```python
from build123d import *

# Parameters (mm, degrees)
SKETCH1_W           = 70
SKETCH1_H           = 50
BOSS_EXTRUDE1_DEPTH = 50
SKETCH2_W           = 20
SKETCH2_H           = 10
CUT_EXTRUDE1_DEPTH  = 50
CUT_EXTRUDE2_DEPTH  = 50
CUT_EXTRUDE3_DEPTH  = 30
SKETCH6_W           = 10
SKETCH6_H           = 10
CUT_EXTRUDE4_DEPTH  = 10
BOSS_EXTRUDE2_DEPTH = 10
CUT_EXTRUDE5_DEPTH  = 10
BOSS_EXTRUDE3_DEPTH = 10
BOSS_EXTRUDE4_DEPTH = 10
BOSS_EXTRUDE5_DEPTH = 10
BOSS_EXTRUDE6_DEPTH = 22


with BuildPart() as part:
    # Sketch1 → Boss-Extrude1 (new body)
    with BuildSketch(Plane.XY):
        with Locations((35, 25)):
            Rectangle(SKETCH1_W, SKETCH1_H)
    extrude(amount=BOSS_EXTRUDE1_DEPTH)

    # Sketch2 → Cut-Extrude1 (cut)
    with BuildSketch(Plane.XY.offset(50)):
        Polygon((0, 20), (30, 50), (0, 50), align=None)
        with Locations((60, 45)):
            Rectangle(SKETCH2_W, SKETCH2_H)
    extrude(amount=-CUT_EXTRUDE1_DEPTH, mode=Mode.SUBTRACT)

    # Sketch3 → Cut-Extrude2 (cut)
    with BuildSketch(Plane.XZ):
        Polygon((0, 10), (20, 20), (20, 50), (0, 50), align=None)
    extrude(amount=-CUT_EXTRUDE2_DEPTH, mode=Mode.SUBTRACT)

    # Sketch5 → Cut-Extrude3 (cut)
    with BuildSketch(Plane.XY.offset(50)):
        Polygon((20, 0), (40, 30), (60, 30), (60, 40), (50, 40), (50, 50), (30, 50), (20, 40), align=None)
    extrude(amount=-CUT_EXTRUDE3_DEPTH, mode=Mode.SUBTRACT)

    # Sketch6 → Cut-Extrude4 (cut)
    with BuildSketch(Plane.XY.offset(50)):
        with Locations((65, 35)):
            Rectangle(SKETCH6_W, SKETCH6_H)
    extrude(amount=-CUT_EXTRUDE4_DEPTH, mode=Mode.SUBTRACT)

    # Sketch7 → Boss-Extrude2 (add)
    with BuildSketch(Plane(origin=(0, 40, 0), x_dir=(1, 0, 0), z_dir=(0, 1, 0))):
        Polygon((60, -40), (0, -10), (60, -10), (60, -20), align=None)
    extrude(amount=-BOSS_EXTRUDE2_DEPTH)

    # Sketch8 → Cut-Extrude5 (cut)
    with BuildSketch(Plane(origin=(0, 0, 10), x_dir=(-1, 0, 0), z_dir=(0, 0, -1))):
        Polygon((0, 30), (-10, 30), (-20, 40), (0, 40), align=None)
    extrude(amount=-CUT_EXTRUDE5_DEPTH, mode=Mode.SUBTRACT)

    # Sketch9 → Boss-Extrude3 (add)
    with BuildSketch(Plane(origin=(0, 40, 0), x_dir=(1, 0, 0), z_dir=(0, 1, 0))):
        Polygon((30, -25), (50, -35), (50, -20), (30, -20), align=None)
    extrude(amount=BOSS_EXTRUDE3_DEPTH)

    # Sketch10 → Boss-Extrude4 (add)
    with BuildSketch(Plane(origin=(-4, 0, 8), x_dir=(0.894427191, 0, 0.447213595), z_dir=(-0.447213595, 0, 0.894427191))):
        Polygon((26.83281573, 40), (38.013155617, 50), (38.013155617, 40), align=None)
    extrude(amount=-BOSS_EXTRUDE4_DEPTH)

    # Sketch11 → Boss-Extrude5 (add)
    with BuildSketch(Plane(origin=(-10, 10, 0), x_dir=(0, 0, 1), z_dir=(-0.707106781, 0.707106781, 0))):
        Polygon((20, 42.426406871), (20, 56.568542495), (25, 56.568542495), align=None)
    extrude(amount=-BOSS_EXTRUDE5_DEPTH)

    # Sketch12 → Boss-Extrude6 (add)
    with BuildSketch(Plane(origin=(-4, 0, 8), x_dir=(0.894427191, 0, 0.447213595), z_dir=(-0.447213595, 0, 0.894427191))):
        Polygon((26.83281573, 0), (26.83281573, 30), (49.193495505, 30), align=None)
    extrude(amount=-BOSS_EXTRUDE6_DEPTH)


solid = part.part
```
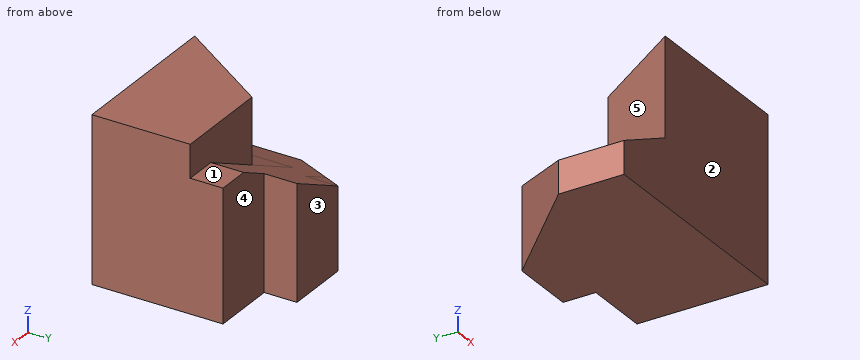
Can you work these out from the model? Positions are in its coordinate system, mm. Face numbers are marked on the shaded views. A direction names the side the tool comes from. Give positions to 0.01 mm unless a question says otherwise; leave off trailing zeros. Loops run counter-clockwise (first coordinate to the right, second up) from the corner with the lowest first, then second, coordinate; pieces in that order, holes last. Notation, with made-up numbers: M 58.25,59 L 79.25,59 A31 cw 79.25,88 Z; hole C 59,45.25 d6. An arc over 180 degrees is marked long. Use CSV: the item, a comma, the result in double quotes. Start each with the question number.
1. Imagine slicing it at D-D, the plane z = 4.5. Write out the boundary of the cut face in (x, y), plus the area to 3 significant figures.
2. Imagine slicing it at C-C, the plane y = 35.5. Write out the boundary of the cut face in (x, z), plus the area to 3 significant figures.
3. If I drill on L1, parallel to Y at x = 53, z = 10.5; L2, parallel to X at y = 18, z = 18; L3, parallel to Y at x = 25.5, z = 41, over which ranges is the centre line in solid material (lowest first)?
4. On a 3-axis mill with a long thin cutter (end or side, diameter ignored), from which of +Z, -Z, +X, -X, +Y, -Y can I reach the whole of each face in a straight line? I mean the marked faces 1, 2, 3, 4 and 5. Say none if no direction works.
5. Imagine slicing it at B-B, the plane x = 59. Write out the boundary of the cut face in (y, z), plus the area to 4 significant figures.
6. Imagine slicing it at A-A, the plane z = 11.5. Write out the boundary of the cut face in (x, y), plus the area to 3 significant figures.
7. For P1, Ø5, axis at y = 44, z = 15.5, coming from the +X side; P2, Ø6, axis at x = 62, z = 18, coming from the +Y side; P3, Ø8, axis at y = 21, z = 15, coming from the -X side, each with a flat end and sliding along its axis, tell me the tip position at first contact or that it passes through.
Response values:
1,outline,"M 0,0 L 70,0 L 70,40 L 50,40 L 50,50 L 30,50 L 0,20 Z"
1,area,"2,850 mm^2"
2,outline,"M 15.5,0 L 70,0 L 70,40 L 60,40 L 15.5,17.75 Z"
2,area,"1,680 mm^2"
3,L1,"0 to 40"
3,L2,"16 to 70"
3,L3,"0 to 8.25"
4,face 1,"+Z, +X, -X, +Y"
4,face 2,"+Z, -Z, +X, -X, -Y"
4,face 3,"+Z, -Z, +X, -X, +Y"
4,face 4,"+Z, -Z, +X, +Y"
4,face 5,"+Z, -X, +Y"
5,outline,"M 0,0 L 40,0 L 40,39.5 L 30,39.5 L 30,50 L 0,50 Z"
5,area,"1,895 mm^2"
6,outline,"M 3,0 L 70,0 L 70,40 L 50,40 L 50,50 L 30,50 L 3,23 Z"
6,area,"2,790 mm^2"
7,P1,"x = 50"
7,P2,"y = 40"
7,P3,"x = 2"
